```python
from build123d import *

# Parameters (mm, degrees)
SKETCH1_R               = 72.5
SKETCH1_R_2             = 3.175
BOSS_EXTRUDE1_DEPTH     = 10
SKETCH8_R               = 8.35
CUT_EXTRUDE4_DEPTH      = 5
SKETCH9_R               = 5.75
CUT_EXTRUDE5_DEPTH      = 1
CUT_EXTRUDE5_DEPTH_BACK = 11
SKETCH10_R              = 72.5
SKETCH10_R_2            = 60.5
SKETCH10_R_3            = 3.175
BOSS_EXTRUDE4_DEPTH     = 20
SKETCH11_W              = 32.27284004
SKETCH11_H              = 12.3
SKETCH11_W_2            = 12.3
SKETCH11_H_2            = 32.27284004
CUT_EXTRUDE6_DEPTH      = 6.45
SKETCH12_R              = 2.15
CUT_EXTRUDE7_DEPTH      = 6


with BuildPart() as part:
    # Sketch1 → Boss-Extrude1 (new body)
    with BuildSketch(Plane(origin=(0, 0, 0), x_dir=(1, 0, 0), z_dir=(0, 1, 0))):
        Circle(SKETCH1_R)
        with Locations((0, 67)):
            Circle(SKETCH1_R_2, mode=Mode.SUBTRACT)
        with Locations((67, 0)):
            Circle(SKETCH1_R_2, mode=Mode.SUBTRACT)
        with Locations((0, -67)):
            Circle(SKETCH1_R_2, mode=Mode.SUBTRACT)
        with Locations((-67, 0)):
            Circle(SKETCH1_R_2, mode=Mode.SUBTRACT)
        with BuildLine():
            Line((10, 17.320508076), (10, 59.667830529))
            ThreePointArc((10, 59.667830529), (30.25, 52.394536929), (46.673857027, 38.494169302))
            Line((46.673857027, 38.494169302), (10, 17.320508076))
        make_face(mode=Mode.SUBTRACT)
        with BuildLine():
            Line((-10, 17.320508076), (-10, 59.667830529))
            ThreePointArc((-10, 59.667830529), (-30.25, 52.394536929), (-46.673857027, 38.494169302))
            Line((-46.673857027, 38.494169302), (-10, 17.320508076))
        make_face(mode=Mode.SUBTRACT)
        with BuildLine():
            Line((-20, 0), (-56.673857027, 21.173661227))
            ThreePointArc((-56.673857027, 21.173661227), (-60.5, 0), (-56.673857027, -21.173661226))
            Line((-56.673857027, -21.173661226), (-20, 0))
        make_face(mode=Mode.SUBTRACT)
        with BuildLine():
            Line((-10, -17.320508076), (-46.673857027, -38.494169302))
            ThreePointArc((-46.673857027, -38.494169302), (-30.25, -52.394536929), (-10, -59.667830529))
            Line((-10, -59.667830529), (-10, -17.320508076))
        make_face(mode=Mode.SUBTRACT)
        with BuildLine():
            Line((10, -17.320508076), (10, -59.667830529))
            ThreePointArc((10, -59.667830529), (30.25, -52.394536929), (46.673857027, -38.494169302))
            Line((46.673857027, -38.494169302), (10, -17.320508076))
        make_face(mode=Mode.SUBTRACT)
        with BuildLine():
            Line((20, 0), (56.673857027, 21.173661227))
            ThreePointArc((56.673857027, 21.173661227), (60.5, 0), (56.673857027, -21.173661226))
            Line((56.673857027, -21.173661226), (20, 0))
        make_face(mode=Mode.SUBTRACT)
    extrude(amount=BOSS_EXTRUDE1_DEPTH)

    # Sketch8 → Cut-Extrude4 (cut)
    with BuildSketch(Plane(origin=(0, 10, 0), x_dir=(1, 0, 0), z_dir=(0, 1, 0))):
        Circle(SKETCH8_R)
    extrude(amount=-CUT_EXTRUDE4_DEPTH, mode=Mode.SUBTRACT)

    # Sketch9 → Cut-Extrude5 (cut, two sides)
    with BuildSketch(Plane(origin=(0, 10, 0), x_dir=(1, 0, 0), z_dir=(0, 1, 0))) as cut_extrude5_sk:
        Circle(SKETCH9_R)
    extrude(amount=CUT_EXTRUDE5_DEPTH, mode=Mode.SUBTRACT)
    extrude(cut_extrude5_sk.sketch, amount=-CUT_EXTRUDE5_DEPTH_BACK, mode=Mode.SUBTRACT)

    # Sketch10 → Boss-Extrude4 (add)
    with BuildSketch(Plane.XZ):
        Circle(SKETCH10_R)
        Circle(SKETCH10_R_2, mode=Mode.SUBTRACT)
        with Locations((0, -67)):
            Circle(SKETCH10_R_3, mode=Mode.SUBTRACT)
        with Locations((-67, 0)):
            Circle(SKETCH10_R_3, mode=Mode.SUBTRACT)
        with Locations((0, 67)):
            Circle(SKETCH10_R_3, mode=Mode.SUBTRACT)
        with Locations((67, 0)):
            Circle(SKETCH10_R_3, mode=Mode.SUBTRACT)
    extrude(amount=BOSS_EXTRUDE4_DEPTH)

    # Sketch11 → Cut-Extrude6 (cut)
    with BuildSketch(Plane.XZ.offset(20)):
        with Locations((-60.5, 0)):
            Rectangle(SKETCH11_W, SKETCH11_H)
        with Locations((0, -60.5)):
            Rectangle(SKETCH11_W_2, SKETCH11_H_2)
        with Locations((0, 60.5)):
            Rectangle(SKETCH11_W_2, SKETCH11_H_2)
        with Locations((60.5, 0)):
            Rectangle(SKETCH11_W, SKETCH11_H)
    extrude(amount=-CUT_EXTRUDE6_DEPTH, mode=Mode.SUBTRACT)

    # Sketch12 → Cut-Extrude7 (cut)
    with BuildSketch(Plane.XZ.offset(20)):
        with Locations((33.5, 58.023702054)):
            Circle(SKETCH12_R)
        with Locations((58.023702054, 33.5)):
            Circle(SKETCH12_R)
        with Locations((33.5, -58.023702054)):
            Circle(SKETCH12_R)
        with Locations((58.023702054, -33.5)):
            Circle(SKETCH12_R)
        with Locations((-58.023702054, -33.5)):
            Circle(SKETCH12_R)
        with Locations((-33.5, -58.023702054)):
            Circle(SKETCH12_R)
        with Locations((-33.5, 58.023702054)):
            Circle(SKETCH12_R)
        with Locations((-58.023702054, 33.5)):
            Circle(SKETCH12_R)
    extrude(amount=-CUT_EXTRUDE7_DEPTH, mode=Mode.SUBTRACT)


solid = part.part
```
Work out the finished part from the listing and answer in its coordinate system (mm). A direction names the side the tool comes from. Give positions to 0.01 mm unless a question says otherwise; leave off trailing zeros. Loops run counter-clockwise (first coordinate to the right, second up) from the corner with the lowest first, then second, coordinate; pieces in that order, holes last. Notation, with made-up numbers: (16.5, -38) -> (60.5, -38) arc R21 ccw to (60.5, -15) -> close; hole circle Ø1 at (1.5, -24.5). An arc over 180 degrees is marked (long way). Write item = value, one per line. Start each with the question number.
(1) Given pin 1 Ø3 at (y, z) = (7, -47) entering from +X; pin 2 Ø11 at (y, z) = (5.5, 30) entering from +X; pin 3 Ø3.5 at (x, z) = (-0.5, 69) entering from -Y, each flat-ended and moving along its own axis, determine where each tip first touches the part or whether it passes through.
(2) Find section D-D on z = -25.5. Give the vertices of the cut face in (x, y).
(3) Which of the six approach directions +Z, -Z, +X, -X, +Y, -Y give full straight-line access (tool end or side, diameter ignored) to faces 3 (the flat face through (66, -17, 6.15)), 4 (the flat face through (-44, -20, 42)), 5 (the flat face through (-13, 0, -1)), 6 (the flat face through (28.594, 4.93, 28.056)), 7 (the flat face through (-6.15, -17, 66))?
(4) Find section B-B on y = 7.5. Give the number of separate pieces and of enclosed holes in the cut face, and give its area (3 significant figures).
(5) Find the intervals of material crossed by probe 1 along X at (y, z) = (3.65, 0) (3 decimals); probe 2 along Z at (x, y) = (0.5, 8.5); probe 3 along X at (y, z) = (6.1, 0) (3 decimals), in increasing order. Write a range as from..to.
(6) The mould has two halves that part along X. Classify faces 1 (the flat face through (-58, -14, -33)), 2 (the flat face through (66, -17, -6.15)): +X half, -X half, draft (parallel to the pull), parting line (faces both ways), or undercut.
(7) Find section A-A on x = 0. Give the vertices of the cut face in (y, z) (3 decimals), and give its area (3 significant figures).
From the geometry:
q1.pin_1 = 56.44
q1.pin_2 = 68.23
q1.pin_3 = -13.55
q2.outline = (-67.87, -20) -> (-54.86, -20) -> (-54.86, 0) -> (-24.17, 0) -> (-24.17, 10) -> (-67.87, 10) -> close; (-10, 0) -> (10, 0) -> (10, 10) -> (-10, 10) -> close; (24.17, 0) -> (54.86, 0) -> (54.86, -20) -> (67.87, -20) -> (67.87, 10) -> (24.17, 10) -> close
q3.face_3 = +X, -X, -Y
q3.face_4 = +Z, -Z, +X, -X, -Y
q3.face_5 = -Y
q3.face_6 = +Y, -Y
q3.face_7 = +Z, -Z, -Y
q4.separate_pieces = 1
q4.enclosed_holes = 11
q4.area = 10,900 mm^2
q5.probe_1 = -72.5..-70.175, -63.825..-60.5, -20..-5.75, 5.75..20, 60.5..63.825, 70.175..72.5
q5.probe_2 = -72.5..-70.14, -63.86..-8.34, 8.34..63.86, 70.14..72.5
q5.probe_3 = -72.5..-70.175, -63.825..-60.5, -20..-8.35, 8.35..20, 60.5..63.825, 70.175..72.5
q6.face_1 = undercut
q6.face_2 = draft
q7.outline = (-13.55, -72.5) -> (10, -72.5) -> (10, -70.175) -> (-13.55, -70.175) -> close; (-13.55, -63.825) -> (10, -63.825) -> (10, -8.35) -> (5, -8.35) -> (5, -5.75) -> (0, -5.75) -> (0, -60.5) -> (-13.55, -60.5) -> close; (-13.55, 60.5) -> (0, 60.5) -> (0, 5.75) -> (5, 5.75) -> (5, 8.35) -> (10, 8.35) -> (10, 63.825) -> (-13.55, 63.825) -> close; (-13.55, 70.175) -> (10, 70.175) -> (10, 72.5) -> (-13.55, 72.5) -> close
q7.area = 1,340 mm^2
